from build123d import *

# Parameters (mm, degrees)
SKETCH1_W             = 50.8
SKETCH1_H             = 152.654
SKETCH1_R             = 3.925
BOSS_EXTRUDE1_DEPTH   = 3.175
F_6_CLEARANCE_HOLE1_D = 3.6576


with BuildPart() as part:
    # Sketch1 → Boss-Extrude1 (new, symmetric)
    with BuildSketch(Plane(origin=(0, 0, 0), x_dir=(0, 0, -1), z_dir=(1, 0, 0))):
        with Locations((-12.7, -63.627)):
            Rectangle(SKETCH1_W, SKETCH1_H)
        Circle(SKETCH1_R, mode=Mode.SUBTRACT)
        with Locations((0, -115.824)):
            Circle(SKETCH1_R, mode=Mode.SUBTRACT)
    extrude(amount=BOSS_EXTRUDE1_DEPTH, both=True)

    # #6 Clearance Hole1 (through all)
    with Locations(Plane.ZY.offset(3.175)):
        with Locations((0, -96.774), (25.4, -96.774), (25.4, -134.874), (0, -134.874)):
            Hole(F_6_CLEARANCE_HOLE1_D / 2)


solid = part.part
CAD build for the part. Positions are in the model's coordinates, mm. Give positions to 0.01 mm unless a question says otherwise; leave off trailing zeros. Write each loop counter-clockwise with the first axis right and the second up, starting at its lowest first coordinate (ties: lowest second). Pieces come first, ordered by that corner, then holes. Notation, with made-up numbers: (0.25, 52) -> (45.25, 52) arc R27 cw to (45.25, 79) -> close; hole circle Ø6 at (19, 63). An arc over 180 degrees is marked (long way). Return JSON: item names as keys, results as strings.
Item 1: Band-saw the part on C-C (y = 0). List the corners of the cut face in (x, z) (3 decimals).
Answer below:
{"outline": "(-3.175, -12.7) -> (3.175, -12.7) -> (3.175, -3.925) -> (-3.175, -3.925) -> close; (-3.175, 3.925) -> (3.175, 3.925) -> (3.175, 38.1) -> (-3.175, 38.1) -> close"}
Item 2: Two-plate mould, pull along Z, no slides. Class faces 1 (the flat face through (0, -139.954, 13)), 2 (the flat face through (0, -65, -12.7)), 3 (the cylindrical face through (-0.044, -112.514, -2.11)): +Z half, -Z half, draft (parallel to the pull), parting line (faces both ways), or undercut.
Answer below:
{"face 1": "draft", "face 2": "-Z half", "face 3": "undercut"}
Item 3: Band-saw the part on B-B (z = 0). List the corners of the cut face in (x, y) (3 decimals).
Answer below:
{"outline": "(-3.175, -139.954) -> (3.175, -139.954) -> (3.175, -136.703) -> (-3.175, -136.703) -> close; (-3.175, -133.045) -> (3.175, -133.045) -> (3.175, -119.749) -> (-3.175, -119.749) -> close; (-3.175, -111.899) -> (3.175, -111.899) -> (3.175, -98.603) -> (-3.175, -98.603) -> close; (-3.175, -94.945) -> (3.175, -94.945) -> (3.175, -3.925) -> (-3.175, -3.925) -> close; (-3.175, 3.925) -> (3.175, 3.925) -> (3.175, 12.7) -> (-3.175, 12.7) -> close"}
Item 4: Drop a flat-ended pin along its axis: pin 1 (7 mm diameter, centred on y = 0, z = 0, fed in from -X). Give the stop position or say it passes through.
Answer below:
{"pin 1": "passes through"}
Item 5: Drill centre lines: probe 1 along Y at (x, z) = (0.75, 0) (3 decimals); probe 2 along Y at (x, z) = (1, 25.4). Where is each one in solid material? Low to high.
Answer below:
{"probe 1": "y = -139.954 to -136.703, -133.045 to -119.749, -111.899 to -98.603, -94.945 to -3.925, 3.925 to 12.7", "probe 2": "y = -139.95 to -136.7, -133.05 to -98.6, -94.95 to 12.7"}
Item 6: Band-saw the part on A-A (z = 25.4). List the corners of the cut face in (x, y) (3 decimals), then the cut area to 3 significant figures.
Answer below:
{"outline": "(-3.175, -139.954) -> (3.175, -139.954) -> (3.175, -136.703) -> (-3.175, -136.703) -> close; (-3.175, -133.045) -> (3.175, -133.045) -> (3.175, -98.603) -> (-3.175, -98.603) -> close; (-3.175, -94.945) -> (3.175, -94.945) -> (3.175, 12.7) -> (-3.175, 12.7) -> close", "area": "923 mm2"}
Item 7: Band-saw the part on D-D (x = 0.25). List the corners of the cut face in (y, z) (3 decimals), then the cut area to 3 significant figures.
Answer below:
{"outline": "(-139.954, -12.7) -> (12.7, -12.7) -> (12.7, 38.1) -> (-139.954, 38.1) -> close; hole circle Ø3.658 at (-134.874, 0); hole circle Ø3.658 at (-134.874, 25.4); hole circle Ø7.85 at (-115.824, 0); hole circle Ø3.658 at (-96.774, 0); hole circle Ø3.658 at (-96.774, 25.4); hole circle Ø7.85 at (0, 0)", "area": "7,620 mm2"}
